from build123d import *

# Parameters (mm, degrees)
EXTRUDE_1_DEPTH     = 3
SKETCH_4_OUTSIDE_W  = 14.556
SKETCH_4_OUTSIDE_H  = 10.656
SKETCH_4_OUTSIDE_R  = 3
CUT_EXTRUDE_1_DEPTH = 1.5
CUT_EXTRUDE_2_DEPTH = 6


with BuildPart() as part:
    # Эскиз1 → Бобышка-Вытянуть1 (new body, symmetric)
    with BuildSketch(Plane.XY):
        Polygon((3, 0), (-3, 0), (-3, -1.5), (-4.95, -1.5), (-4.95, -6.5), (4.95, -6.5), (4.95, -1.5), (3, -1.5), align=None)
    extrude(amount=EXTRUDE_1_DEPTH, both=True)

    # Эскиз3 → Отверстие обработанное метчиком M51 (revolve, cut)
    with BuildSketch(Plane(origin=(0, 0, 0), x_dir=(0, 0, 1), z_dir=(1, 0, 0))):
        Polygon((0, 0), (0, 6.5), (2.6, 6.5), (2.1, 6), (2.1, 0.5), (2.6, 0), align=None)
    revolve(axis=Axis((0, 6.35, 0), (0, -1, 0)), mode=Mode.SUBTRACT)

    # Эскиз4 outside → Вырез-Вытянуть1 (cut)
    with BuildSketch(Plane(origin=(0, 0, 0), x_dir=(1, 0, 0), z_dir=(0, 1, 0))):
        Rectangle(SKETCH_4_OUTSIDE_W, SKETCH_4_OUTSIDE_H)
        with Locations(Location((0, 0, 0), (0, 0, 270))):  # turned: the seam where the file's is
            Circle(SKETCH_4_OUTSIDE_R, mode=Mode.SUBTRACT)
    extrude(amount=-CUT_EXTRUDE_1_DEPTH, mode=Mode.SUBTRACT)

    # Эскиз5 → Вырез-Вытянуть2 (cut, through all)
    with BuildSketch(Plane(origin=(0, -1.5, 0), x_dir=(1, 0, 0), z_dir=(0, 1, 0))):
        with BuildLine():
            Line((-4.95, 0), (-4.95, 3))
            Line((-4.95, 3), (-3.937321425, 3))
            ThreePointArc((-3.937321425, 3), (-4.690002188, 1.583154912), (-4.95, 0))
        make_face()
        with BuildLine():
            Line((4.95, 0), (4.95, -3))
            Line((4.95, -3), (3.937321425, -3))
            ThreePointArc((3.937321425, -3), (4.690002188, -1.583154912), (4.95, 0))
        make_face()
    extrude(amount=-CUT_EXTRUDE_2_DEPTH, mode=Mode.SUBTRACT)

    # Вырез-По траектории1: sweep along a path in Эскиз7
    with BuildLine(Plane.XZ.offset(6.5)) as sweep_1_path:
        Line((0, 4.95), (-4.95, 4.95))
        Line((-4.95, 4.95), (-4.95, 0))
        ThreePointArc((-4.95, 0), (-3.500178567, -3.500178567), (0, -4.95))
        Line((0, -4.95), (4.95, -4.95))
        Line((4.95, -4.95), (4.95, 0))
        ThreePointArc((4.95, 0), (3.500178567, 3.500178567), (0, 4.95))
    # Эскиз6 → Вырез-По траектории1 (sweep, cut)
    with BuildSketch(Plane.XY.offset(3)):
        Polygon((-4.95, -3), (-4.95, -6.5), (-3, -6.5), align=None)
    sweep(path=sweep_1_path.line, transition=Transition.RIGHT, mode=Mode.SUBTRACT)


solid = part.part
The listing builds one solid part. Answer for the finished solid, in the listing's coordinates (mm). A direction names the side the tool comes from. Round coordinates to 2 decimals unless told otherwise and drop trailing zeros. Write each loop counter-clockwise with the first axis right and the second up, starting at its lowest first coordinate (ties: lowest second). Pieces come first, ordered by that corner, then holes. Notation, with made-up numbers: (34, 83.5) - (40, 83.5) arc R22 cw to (40, 111.5) - close; hole circle Ø1 at (67.25, 88). An arc over 180 degrees is marked (long way). Use one line per item in the form item = value. Start each with the question number.
Item 1: A flat-ended cylindrical pin translates along its axis: pin 1 Ø1.5 at (x, z) = (-1.5, -1) entering from +Y. Find the tip coordinate at first contact, or state that the pin passes through.
Item 2: Determine the mould class of faces 1 (the cylindrical face through (0.9, -0.74, 2.86)), 2 (the cylindrical face through (-0.631, -3.212, 2.003)), 3 (the flat face through (-4.95, -2, 2)) for opening direction X: +X half, -X half, draft (parallel to the pull), parting line (faces both ways), or undercut.
Item 3: A tool of negligible diameter and unlimited length cuts with its end or side. For faces 4 (the flat face through (-1, -3, 3)), 5 (the flat face through (4, -1.5, 0)), from which of +Z, -Z, +X, -X, +Y, -Y can it reach the whole face along a straight path? Write none if from no direction.
Item 4: Find the intervals of material crossed by line 1 (X direction, y = -1.8, z = 0); line 2 (Z direction, x = 0, y = -3.2); line 3 (Z direction, x = 1.25, y = -3), in increasing order. Write a range as [from, to].
Item 5: A cutting plane is placed at A-A (y = -5.25). Write down the section's boundary in (x, z), plus the area to 3 significant figures.
The answers:
q1.pin_1 = -0.05
q2.face_1 = parting line
q2.face_2 = undercut
q2.face_3 = -X half
q3.face_4 = +Z, +X, -X, +Y, -Y
q3.face_5 = +X, +Y
q4.line_1 = [-4.95, -2.1], [2.1, 4.95]
q4.line_2 = [-3, -2.1], [2.1, 3]
q4.line_3 = [-3, -1.69], [1.69, 3]
q5.outline = (-3.7, 0) arc R3.7 ccw to (-2.16, -3) - (3.7, -3) - (3.7, 0) arc R3.7 ccw to (2.16, 3) - (-3.7, 3) - close; hole circle Ø4.2 at (0, 0)
q5.area = 27.7 mm^2
